from build123d import *

# Parameters (mm, degrees)
SKETCH_1_R          = 1.6
EXTRUDE_1_DEPTH     = 3
FILLET_1_R          = 10
SKETCH_2_R          = 1
CUT_EXTRUDE_1_DEPTH = 3


with BuildPart() as part:
    # 草图1 → 凸台-拉伸1 (new body)
    with BuildSketch(Plane(origin=(0, 0, 0), x_dir=(1, 0, 0), z_dir=(0, 1, 0))):
        Polygon((-10, 25), (-10, 15), (10, 15), (10, 25), (20, 25), (20, -25), (-20, -25), (-20, 25), align=None)
        with Locations(Location((-15, 20, 0), (0, 0, 270))):
            Circle(SKETCH_1_R, mode=Mode.SUBTRACT)
        with Locations(Location((15, 20, 0), (0, 0, 270))):
            Circle(SKETCH_1_R, mode=Mode.SUBTRACT)
        with BuildLine():
            Line((4.1, 10), (4.1, -18))
            ThreePointArc((4.1, -18), (0, -22.1), (-4.1, -18))
            Line((-4.1, -18), (-4.1, 10))
            ThreePointArc((-4.1, 10), (0, 14.1), (4.1, 10))
        make_face(mode=Mode.SUBTRACT)
    extrude(amount=EXTRUDE_1_DEPTH)

    # 圆角1
    fillet_1_edges = [part.edges().sort_by_distance(p)[0] for p in [
        (20, 1.5, 25),
        (-20, 1.5, 25),
    ]]
    fillet(fillet_1_edges, radius=FILLET_1_R)

    # 草图2 → 切除-拉伸1 (cut)
    with BuildSketch(Plane(origin=(0, 3, 0), x_dir=(1, 0, 0), z_dir=(0, 1, 0))):
        with Locations((-10, 15)):
            Circle(SKETCH_2_R)
        with Locations((10, 15)):
            Circle(SKETCH_2_R)
    extrude(amount=-CUT_EXTRUDE_1_DEPTH, mode=Mode.SUBTRACT)


solid = part.part
Model file for the job. Use its own axes, mm. A direction names the side the tool comes from. Give positions to 0.01 mm unless a question says otherwise; leave off trailing zeros. Loops run counter-clockwise (first coordinate to the right, second up) from the corner with the lowest first, then second, coordinate; pieces in that order, holes last.
Item 1: Slice it at C-C (z = 21). Write the cut outline in (x, y), plus the area to 3 significant figures.
Check values:
outline: (-18, 0) - (-2.79, 0) - (-2.79, 3) - (-18, 3) - close; (2.79, 0) - (18, 0) - (18, 3) - (2.79, 3) - close
area: 91.2 mm2
Item 2: Mould opens along X. For faces 1 (the face through (5, 0, 0)), 2 (the face through (0.1, 1.5, 22.1)), 3 (the face through (-17.15, 1.52, 21.99)), 4 (the face through (-4.1, 1, 4)) say: +X half, -X half, draft (parallel to the pull), parting line (faces both ways), or undercut.
Check values:
face 1: draft
face 2: undercut
face 3: -X half
face 4: undercut
Item 3: Slice it at D-D (x = 6). Write the cut outline in (y, z).
Check values:
outline: (0, -15) - (3, -15) - (3, 25) - (0, 25) - close
Item 4: Drop a flat-ended pin along its axis: P1, Ø1.8, axis at x = 10, z = -15, coming from the -Y side. Give the stop position or say it passes through.
Check values:
P1: passes through
Item 5: Which spindle directions (+Z, -Z, +X, -X, +Y, -Y) get a long thin tool onto all of the face, cutting with end or side? Do faces 5 (the face through (4.1, 1, 4)), 6 (the face through (16.99, 1.52, 22.15)), 7 (the face through (10, 1, -20)). Say none if no direction does.
Check values:
face 5: +Y, -Y
face 6: +Z, +X, +Y, -Y
face 7: -Z, +Y, -Y
Item 6: Drill centre lines: line 1 along X through (y, z) = (1.7, -20); line 2 along X through (y, z) = (2.05, -8); line 3 along X through (y, z) = (1.9, -17). Where is each one in solid material? Low to high.
Check values:
line 1: x = -20 to -16.6, -13.4 to -10, 10 to 13.4, 16.6 to 20
line 2: x = -20 to -4.1, 4.1 to 20
line 3: x = -20 to -10, 10 to 20
Item 7: Slice it at B-B (y = 0.8). Write the cut outline in (x, z), plus the area to 3 significant figures.
Check values:
outline: (-20, -25) - (-10, -25) - (-10, -16) arc R1 cw (long way) to (-9, -15) - (9, -15) arc R1 cw (long way) to (10, -16) - (10, -25) - (20, -25) - (20, 15) arc R10 ccw to (10, 25) - (-10, 25) arc R10 ccw to (-20, 15) - close; hole circle Ø3.2 at (-15, -20); hole (-4.1, -10) arc R4.1 ccw to (4.1, -10) - (4.1, 18) arc R4.1 ccw to (-4.1, 18) - close; hole circle Ø3.2 at (15, -20)
area: 1,450 mm2
Item 8: Slice it at A-A (x = 0). Write the cut outline in (y, z).
Check values:
outline: (0, -15) - (3, -15) - (3, -14.1) - (0, -14.1) - close; (0, 22.1) - (3, 22.1) - (3, 25) - (0, 25) - close
